Can you work these out from the model? Positions are in its coordinate system, mm. A direction names the side the tool comes from. Round coordinates to 2 decimals unless told otherwise and drop trailing zeros. Loops run counter-clockwise (first coordinate to the right, second up) from the corner with the lowest first, then second, coordinate; pieces in that order, holes last.
from build123d import *
from build123d.topology import SkipClean

# Parameters (mm, degrees)
SKIZZE1_R                       = 15
AUFSATZ_LINEAR_AUSTRAGEN1_DEPTH = 5
AUFSATZ_LINEAR_START            = 4
SKIZZE2_R                       = 15
SKIZZE2_R_2                     = 13
AUFSATZ_LINEAR_AUSTRAGEN2_DEPTH = 4
AUFSATZ_LINEAR_AUSTRAGEN3_DEPTH = 2
AUFSATZ_LINEAR_START_2          = 3
AUFSATZ_LINEAR_AUSTRAGEN6_DEPTH = 3
SKIZZE12_R                      = 2
SCHNITT_LINEAR_AUSTRAGEN1_DEPTH = 10
SKIZZE13_R                      = 3.5
SCHNITT_LINEAR_AUSTRAGEN2_DEPTH = 7
AUFSATZ_LINEAR_AUSTRAGEN7_DEPTH = 9
SKIZZE15_R                      = 3.5
SKIZZE15_R_2                    = 2
AUFSATZ_LINEAR_AUSTRAGEN8_DEPTH = 2


with BuildPart() as part:
    # Skizze1 → Aufsatz-Linear austragen1 (new body)
    with BuildSketch(Plane(origin=(0, 0, 0), x_dir=(1, 0, 0), z_dir=(0, 1, 0))):
        with Locations(Location((0, 0, 0), (0, 0, 270))):
            Circle(SKIZZE1_R)
    extrude(amount=-AUFSATZ_LINEAR_AUSTRAGEN1_DEPTH)

    # Skizze2 → Aufsatz-Linear austragen2 (add)
    with BuildSketch(Plane(origin=(0, 0, 0), x_dir=(1, 0, 0), z_dir=(0, 1, 0)).offset(AUFSATZ_LINEAR_START)):
        with Locations(Location((0, 0, 0), (0, 0, 270))):
            Circle(SKIZZE2_R)
        with Locations(Location((0, 0, 0), (0, 0, 270))):
            Circle(SKIZZE2_R_2, mode=Mode.SUBTRACT)
    extrude(amount=-AUFSATZ_LINEAR_AUSTRAGEN2_DEPTH)

    # Skizze3 → Aufsatz-Linear austragen3 (add)
    with BuildSketch(Plane(origin=(0, 4, 0), x_dir=(1, 0, 0), z_dir=(0, 1, 0))):
        with BuildLine():
            Line((-6.042078, -7.968268), (-7.854702, -10.358748))
            ThreePointArc((-7.854702, -10.358748), (-12.566291, -3.329914), (-11.953671, 5.109771))
            Line((-11.953671, 5.109771), (-9.195131, 3.930593))
            ThreePointArc((-9.195131, 3.930593), (-9.666378, -2.561472), (-6.042078, -7.968268))
        make_face()
        with BuildLine():
            Line((6.042078, 7.968268), (7.854702, 10.358748))
            ThreePointArc((7.854702, 10.358748), (12.566291, 3.329914), (11.953671, -5.109771))
            Line((11.953671, -5.109771), (9.195131, -3.930593))
            ThreePointArc((9.195131, -3.930593), (9.666378, 2.561472), (6.042078, 7.968268))
        make_face()
    extrude(amount=-AUFSATZ_LINEAR_AUSTRAGEN3_DEPTH)

    # Skizze11 → Aufsatz-Linear austragen6 (add)
    with BuildSketch(Plane(origin=(0, 0, 0), x_dir=(1, 0, 0), z_dir=(0, 1, 0)).offset(AUFSATZ_LINEAR_START_2)):
        with BuildLine():
            Line((-9.195131, 3.930593), (-9.654888, 4.127123))
            ThreePointArc((-9.654888, 4.127123), (-10.457571, 0.942977), (-10.237444, -2.333398))
            Line((-10.237444, -2.333398), (-9.755374, -2.198334))
            ThreePointArc((-9.755374, -2.198334), (-9.958481, 0.910302), (-9.195131, 3.930593))
        make_face()
        with BuildLine():
            Line((-9.512352, -3.084666), (-9.96953, -3.295219))
            ThreePointArc((-9.96953, -3.295219), (-8.541911, -6.106207), (-6.344182, -8.366681))
            Line((-6.344182, -8.366681), (-6.042078, -7.968268))
            ThreePointArc((-6.042078, -7.968268), (-8.151532, -5.792455), (-9.512352, -3.084666))
        make_face()
        with BuildLine():
            Line((6.344182, 8.366681), (6.042078, 7.968268))
            ThreePointArc((6.042078, 7.968268), (7.872714, 6.166066), (9.183817, 3.956957))
            Line((9.183817, 3.956957), (9.638169, 4.166018))
            ThreePointArc((9.638169, 4.166018), (8.262583, 6.479176), (6.344182, 8.366681))
        make_face()
        with BuildLine():
            Line((10.078818, 2.944049), (9.595423, 2.815647))
            ThreePointArc((9.595423, 2.815647), (9.982443, -0.592313), (9.195131, -3.930593))
            Line((9.195131, -3.930593), (9.654888, -4.127123))
            ThreePointArc((9.654888, -4.127123), (10.481181, -0.628367), (10.078818, 2.944049))
        make_face()
    extrude(amount=-AUFSATZ_LINEAR_AUSTRAGEN6_DEPTH)

    # Skizze12 → Schnitt-Linear austragen1 (cut)
    with BuildSketch(Plane(origin=(0, 0, 0), x_dir=(1, 0, 0), z_dir=(0, 1, 0))):
        with Locations(Location((0, 6.5, 0), (0, 0, 270))):
            Circle(SKIZZE12_R)
        with Locations((0, 14)):
            Circle(SKIZZE12_R)
    extrude(amount=-SCHNITT_LINEAR_AUSTRAGEN1_DEPTH, mode=Mode.SUBTRACT)

    # Skizze13 → Schnitt-Linear austragen2 (cut)
    with BuildSketch(Plane(origin=(0, 4, 0), x_dir=(1, 0, 0), z_dir=(0, 1, 0))):
        with Locations((0, 14)):
            Circle(SKIZZE13_R)
        with Locations(Location((0, 6.5, 0), (0, 0, 270))):
            Circle(SKIZZE13_R)
    extrude(amount=-SCHNITT_LINEAR_AUSTRAGEN2_DEPTH, mode=Mode.SUBTRACT)

    # Skizze14 → Aufsatz-Linear austragen7 (add)
    with SkipClean():  # the faces are left unmerged after this step: merging them gives an invalid solid
        with BuildSketch(Plane(origin=(0, 4, 0), x_dir=(1, 0, 0), z_dir=(0, 1, 0))):
            with BuildLine():
                Line((-5.994789, 13.75), (-3.448498, 14.598214))
                ThreePointArc((-3.448498, 14.598214), (0, 17.5), (3.448498, 14.598214))
                Line((3.448498, 14.598214), (5.994789, 13.75))
                ThreePointArc((5.994789, 13.75), (4.330127, 18.153312), (0, 20))
                ThreePointArc((0, 20), (-4.330127, 18.153312), (-5.994789, 13.75))
            make_face()
        extrude(amount=-AUFSATZ_LINEAR_AUSTRAGEN7_DEPTH)

    # Skizze15 → Aufsatz-Linear austragen8 (add)
    with BuildSketch(Plane(origin=(0, -3, 0), x_dir=(1, 0, 0), z_dir=(0, 1, 0))):
        with Locations(Location((0, 14, 0), (0, 0, 270))):
            Circle(SKIZZE15_R)
        with Locations(Location((0, 14, 0), (0, 0, 270))):
            Circle(SKIZZE15_R_2, mode=Mode.SUBTRACT)
    extrude(amount=-AUFSATZ_LINEAR_AUSTRAGEN8_DEPTH)


solid = part.part
(1) If we section it at D-D, the plane x = 11: List the corners of the cut face in (y, z) for me, then the cut area to 3 significant figures.
Worked answers:
outline: (-5, -10.2) - (4, -10.2) - (4, 4.7) - (2, 4.7) - (2, -6.93) - (0, -6.93) - (0, 6.93) - (4, 6.93) - (4, 10.2) - (-5, 10.2) - close
area: 151 mm2
(2) If we section it at A-A, the plane z = -5.5: List the corners of the cut face in (x, y) for me, then the cut area to 3 significant figures.
Worked answers:
outline: (-13.96, -5) - (-1.73, -5) - (-1.73, -3) - (-3.35, -3) - (-3.35, 0) - (-11.78, 0) - (-11.78, 4) - (-13.96, 4) - close; (1.73, -5) - (13.96, -5) - (13.96, 4) - (8.35, 4) - (8.35, 0) - (3.35, 0) - (3.35, -3) - (1.73, -3) - close; hole (8.94, 0) - (11.78, 0) - (11.78, 2) - (8.94, 2) - close
area: 138 mm2
(3) If we mould it in two halves opening along Y, with no side actions, what happens to faces 1 (the cylindrical face through (-8.57, 1.01, 6.07)), 2 (the flat face through (2, -3, -12)), 3 (the cylindrical face through (8, 1, -6))? For each: released by +Y, released by -Y, zero draft, split by the parting line, or undercut.
Worked answers:
face 1: undercut
face 2: released by +Y
face 3: zero draft
(4) If we section it at B-B, the plane y = 1: List the corners of the cut face in (x, z) for me.
Worked answers:
outline: (-10.24, 2.33) arc R10.5 ccw to (-9.65, -4.13) - (-9.2, -3.93) arc R10 cw to (-9.76, 2.2) - close; (-9.97, 3.3) - (-9.51, 3.08) arc R10 cw to (-6.04, 7.97) - (-6.34, 8.37) arc R10.5 ccw to start; (-5.99, -13.75) arc R6 ccw (long way) to (5.99, -13.75) arc R15 ccw (long way) to start; (6.04, -7.97) - (6.34, -8.37) arc R10.5 ccw to (9.64, -4.17) - (9.18, -3.96) arc R10 cw to start; (9.2, 3.93) arc R10 cw to (9.6, -2.82) - (10.08, -2.94) arc R10.5 ccw to (9.65, 4.13) - close; hole (-3.21, -12.6) arc R3.5 ccw (long way) to (3.21, -12.6) arc R13 ccw (long way) to start
(5) For faces 4 (the flat face through (-2, -3, -5)), 5 (the flat face through (10.5, 2, -2.7)), 6 (the cylindrical face through (0, -4, -12)), which set-ups out of +Z, -Z, +X, -X, +Y, -Y let a thin tool reach every point of the face, with its end or its side?
Worked answers:
face 4: +Y
face 5: none
face 6: +Y, -Y
(6) If we section it at C-C, the plane z = 0: List the corners of the cut face in (x, y) for me, then the cut area to 3 significant figures.
Worked answers:
outline: (-15, -5) - (15, -5) - (15, 4) - (10, 4) - (10, 0) - (-10, 0) - (-10, 4) - (-15, 4) - close; hole (-13, 0) - (-10.5, 0) - (-10.5, 2) - (-13, 2) - close; hole (10.5, 0) - (13, 0) - (13, 2) - (10.5, 2) - close
area: 180 mm2
(7) Will these pins go through, and if not, where does the flat tip stop? P1, Ø3, axis at x = -8, z = -2.5, coming from the +Y side; P2, Ø1.5, axis at x = 3.5, y = -2.5, coming from the +Z side; P3, Ø6.5, axis at x = 0, z = -14, coming from the +Y side.
Worked answers:
P1: stops at y = 0
P2: stops at z = 14.75
P3: stops at y = -3
(8) If I drill on line 1 (X direction, y = -4.1, z = -14); line 2 (X direction, y = -1.25, z = -14); line 3 (X direction, y = 1.5, z = -0.5), over which ranges is the centre line in solid material (lowest first)?
Worked answers:
line 1: x = -6 to -2, 2 to 6
line 2: x = -6 to -3.5, 3.5 to 6
line 3: x = -14.99 to -12.99, -10.49 to -9.99, 9.99 to 10.49, 12.99 to 14.99
